```python
from build123d import *

# Parameters (mm, degrees)
SKETCH1_R               = 2.85
BOSS_EXTRUDE1_DEPTH     = 40
SKETCH2_R               = 4
BOSS_EXTRUDE2_DEPTH     = 5
CUT_EXTRUDE1_DEPTH      = 10
CUT_EXTRUDE1_DEPTH_BACK = 10
SKETCH3_W               = 2.5
SKETCH3_H               = 8


with BuildPart() as part:
    # Sketch1 → Boss-Extrude1 (new body)
    with BuildSketch(Plane.XY):
        Circle(SKETCH1_R)
    extrude(amount=BOSS_EXTRUDE1_DEPTH)

    # Sketch2 → Boss-Extrude2 (add)
    with BuildSketch(Plane(origin=(0, 0, 0), x_dir=(-1, 0, 0), z_dir=(0, 0, -1))):
        Circle(SKETCH2_R)
    extrude(amount=BOSS_EXTRUDE2_DEPTH)

    # Sketch3 → Cut-Extrude1 (cut, two sides: drawn at the far end of the back side and taken through both)
    with BuildSketch(Plane(origin=(0, 0, 0), x_dir=(0, 0, -1), z_dir=(1, 0, 0)).offset(-CUT_EXTRUDE1_DEPTH_BACK)):
        with Locations((3.75, 0)):
            Rectangle(SKETCH3_W, SKETCH3_H)
    extrude(amount=CUT_EXTRUDE1_DEPTH + CUT_EXTRUDE1_DEPTH_BACK, mode=Mode.SUBTRACT)


solid = part.part
```
Geometry check sheet. Reference: the model listing, model coordinates, mm. A direction names the side the tool comes from. Give positions to 0.01 mm unless a question says otherwise; leave off trailing zeros. Order: outer loops, then holes, each group sorted by start corner. A loop starts at its lowest first (then second) coordinate and runs counter-clockwise, first axis right, second up. Notation, with made-up numbers: (35, -40) - (88, -40) arc R18 cw to (88, -30) - close; hole circle Ø9 at (17.25, 17.5). An arc over 180 degrees is marked (long way). Answer in a Markdown table with one row per item. Add a question column.
Q1. Cross-section at B-B, the plane y = 0. Enter the section's corners in (x, z).
Q2. Cross-section at C-C, the plane z = 31. Enter the section's corners in (x, y).
Q3. Material ranges on probe 1 along Z at (x, y) = (-0.5, 3.5); probe 2 along Y at (x, z) = (0.5, 2.5); probe 3 along X at (y, z) = (0.75, 22.5), recorded low to high. Write a range as from..to.
Q4. Cross-section at D-D, the plane y = 3.5. Enter the section's corners in (x, z), then the cut area to 3 significant figures.
Q5. Tool access check on faces 1 (the flat face through (1, 3, 0)), 2 (the flat face through (0, 0, -2.5)). Record the directions out of +Z, -Z, +X, -X, +Y, -Y that give a thin tool (end or side, any length) a straight path to the whole face; none if there is none.
Q6. Cross-section at A-A, the plane x = 2. Enter the section's corners in (y, z), then the cut area to 3 significant figures.
Q7. Gauge pin test, flat ends, axial feed: pin 1 (4 mm diameter, centred on x = -0.5, z = 35.5, fed in from -Y); pin 2 (4 mm diameter, centred on x = -3, z = 20.5, fed in from -Y); pin 3 (3 mm diameter, centred on x = -3, z = 6.5, fed in from -Y). Record the tip position at first contact, or that the pin passes through.
Check values:
| question | item | result |
|---|---|---|
| 1 | outline | (-4, -2.5) - (4, -2.5) - (4, 0) - (2.85, 0) - (2.85, 40) - (-2.85, 40) - (-2.85, 0) - (-4, 0) - close |
| 2 | outline | circle Ø5.7 at (0, 0) |
| 3 | probe 1 | z = -2.5..0 |
| 3 | probe 2 | y = -2.81..2.81 |
| 3 | probe 3 | x = -2.75..2.75 |
| 4 | outline | (-1.94, -2.5) - (1.94, -2.5) - (1.94, 0) - (-1.94, 0) - close |
| 4 | area | 9.68 mm^2 |
| 5 | face 1 | +Z |
| 5 | face 2 | -Z, +X, -X, +Y, -Y |
| 6 | outline | (-3.46, -2.5) - (3.46, -2.5) - (3.46, 0) - (2.03, 0) - (2.03, 40) - (-2.03, 40) - (-2.03, 0) - (-3.46, 0) - close |
| 6 | area | 180 mm^2 |
| 7 | pin 1 | stops at y = -2.85 |
| 7 | pin 2 | stops at y = -2.67 |
| 7 | pin 3 | stops at y = -2.42 |
